The drawing under review shows one solid part. Ordinate dimensions are in mm from its lowest x, y, z. A direction names the side the tool comes from. Round coordinates to 2 decimals unless told otherwise and drop trailing zeros. Write each loop counter-clockwise with the first axis right and the second up, starting at its lowest first coordinate (ties: lowest second). Pieces come first, ordered by that corner, then holes. Notation, with made-up numbers: (72.25, 44.25) -> (101.25, 44.25) arc R7 cw to (101.25, 53.25) -> close; hole circle Ø11 at (60.5, -35). An arc over 180 degrees is marked (long way). Write item = value, one per line. Start each with the question number.
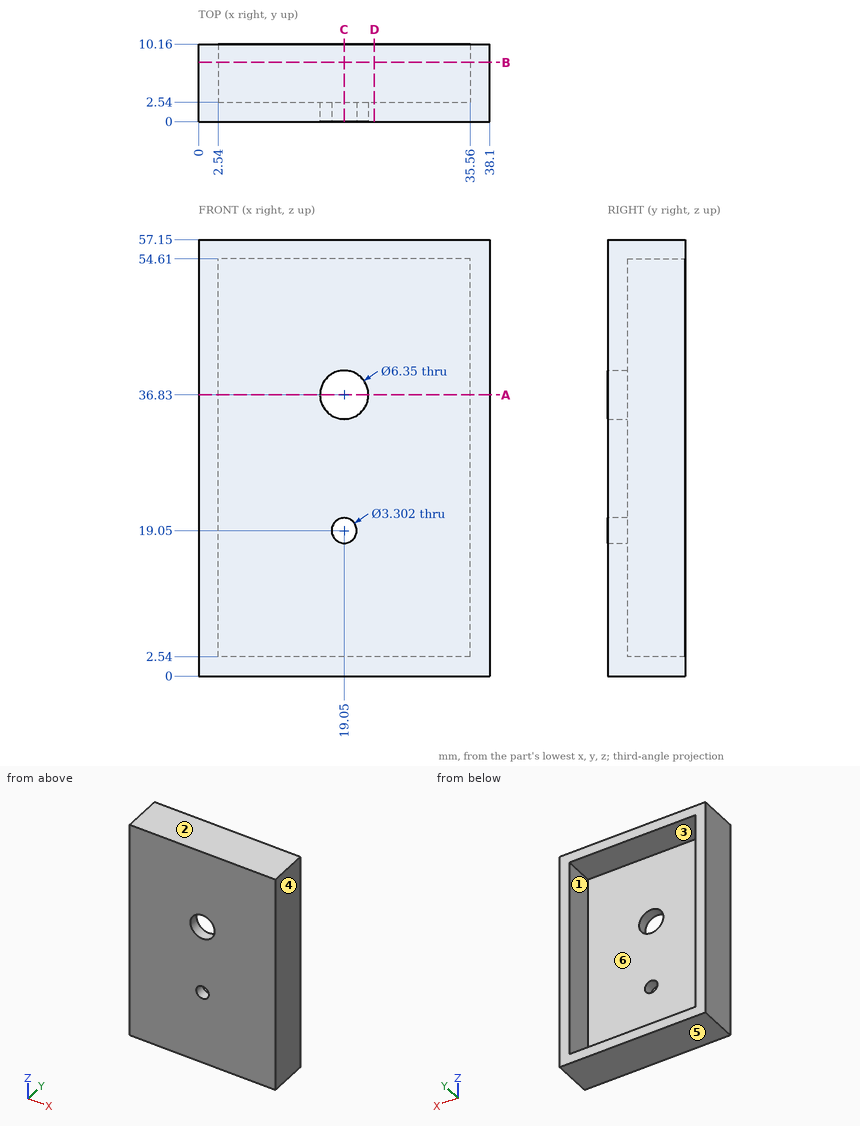
1. Draft analysis for pull direction Z (two halves, no side actions). For the marked faces 1, 2, 3 and 4, state which applies: +Z half, -Z half, draft (parallel to the pull), parting line (faces both ways), or undercut.
2. Consider section C-C, the plane x = 19.05. Give the boundary of the cut face in (y, z) (3 decimals).
3. Clearance check with a flat-ended pin moving along its axis: pin 1 Ø10 at (x, z) = (20.5, 39.5) entering from +Y. State where the tip first meets the part, or that it passes through.
4. Consider section D-D, the plane x = 23. Give the boundary of the cut face in (y, z).
5. Wall thickness on L1, parallel to Z at x = 33.5, y = 9.5; L2, parallel to X at y = 7.5, z = 47.5; L3, parallel to Z at x = 18, y = 0.75: over which ranges is each line inside the solid? List them lowest first. Write a range as from..to.
6. Consider section A-A, the plane z = 36.83. Give the boundary of the cut face in (x, y) (3 decimals).
7. Consider section B-B, the plane y = 7.75. Give the boundary of the cut face in (x, z), then the cut area to 3 significant figures.
8. Machinability: for the marked faces 5 and 6, which of the approach directions +Z, -Z, +X, -X, +Y, -Y give a long, thin tool a straight path to every point of the face, cutting with its end or side? Answer none if there is none.
Outcome:
q1.face_1 = undercut
q1.face_2 = +Z half
q1.face_3 = undercut
q1.face_4 = draft
q2.outline = (0, 0) -> (10.16, 0) -> (10.16, 2.54) -> (2.54, 2.54) -> (2.54, 17.399) -> (0, 17.399) -> close; (0, 20.701) -> (2.54, 20.701) -> (2.54, 33.655) -> (0, 33.655) -> close; (0, 40.005) -> (2.54, 40.005) -> (2.54, 54.61) -> (10.16, 54.61) -> (10.16, 57.15) -> (0, 57.15) -> close
q3.pin_1 = 2.54
q4.outline = (0, 0) -> (10.16, 0) -> (10.16, 2.54) -> (2.54, 2.54) -> (2.54, 54.61) -> (10.16, 54.61) -> (10.16, 57.15) -> (0, 57.15) -> close
q5.L1 = 0..2.54, 54.61..57.15
q5.L2 = 0..2.54, 35.56..38.1
q5.L3 = 0..17.78, 20.32..33.83, 39.83..57.15
q6.outline = (0, 0) -> (15.875, 0) -> (15.875, 2.54) -> (2.54, 2.54) -> (2.54, 10.16) -> (0, 10.16) -> close; (22.225, 0) -> (38.1, 0) -> (38.1, 10.16) -> (35.56, 10.16) -> (35.56, 2.54) -> (22.225, 2.54) -> close
q7.outline = (0, 0) -> (38.1, 0) -> (38.1, 57.15) -> (0, 57.15) -> close; hole (2.54, 2.54) -> (35.56, 2.54) -> (35.56, 54.61) -> (2.54, 54.61) -> close
q7.area = 458 mm2
q8.face_5 = -Z, +X, -X, +Y, -Y
q8.face_6 = +Y
